```python
from build123d import *

# Parameters (mm, degrees)
F0_W     = 50.800353
F0_H     = 44.45
F1_DEPTH = 5


# Not quite as in the source:
# - ends of sketch curves that miss each other by under 0.0002 mm in the source are joined


with BuildPart() as f1:
    # F0 (on Front) → F1 (new body)
    with BuildSketch(Plane.XZ):
        with Locations((5e-07, 0)):
            Rectangle(F0_W, F0_H)
        with BuildLine():
            add(Edge.make_bspline(
                [(-7.08854, -11.336161), (-7.08854, -10.361789), (-7.878409, -9.572272), (-8.852429, -9.572272)],
                knots=[0, 0, 0, 0, 1, 1, 1, 1], degree=3))
            Line((-7.08854, -11.336161), (-7.08854, -15.052322))
            add(Edge.make_bspline(
                [(-8.852429, -16.816211), (-7.878409, -16.816211), (-7.08854, -16.026695), (-7.08854, -15.052322)],
                knots=[0, 0, 0, 0, 1, 1, 1, 1], degree=3))
            Line((-8.852429, -16.816211), (-16.378237, -16.816211))
            add(Edge.make_bspline(
                [(-18.142126, -15.052322), (-18.142126, -16.026695), (-17.352257, -16.816211), (-16.378237, -16.816211)],
                knots=[0, 0, 0, 0, 1, 1, 1, 1], degree=3))
            Line((-18.142126, -15.052322), (-18.142126, -11.336161))
            add(Edge.make_bspline(
                [(-16.378237, -9.572272), (-17.352257, -9.572272), (-18.142126, -10.361789), (-18.142126, -11.336161)],
                knots=[0, 0, 0, 0, 1, 1, 1, 1], degree=3))
            Line((-16.378237, -9.572272), (-8.852429, -9.572272))
        make_face(mode=Mode.SUBTRACT)
        with BuildLine():
            Line((-1.5500305536, -19.2250000002), (-1.5500305536, -8.1871465892))
            ThreePointArc((-1.5500305536, -8.1871465892), (-1.5500734508, -8.1804888446), (-1.55008775, -8.1738309772))
            ThreePointArc((-1.55008775, -8.1738309772), (-9.17611e-05, -6.6238309772), (1.54991225, -8.173822955))
            Line((1.54991225, -8.173822955), (1.5499694464, -19.224991978))
            ThreePointArc((1.5499694464, -19.224991978), (-2.65425e-05, -20.7749959891), (-1.5500305536, -19.2250000002))
        make_face(mode=Mode.SUBTRACT)
        with BuildLine():
            add(Edge.make_bspline(
                [(-0.0001188036, 5.1738309774), (-2.8576188036, 5.1738309774), (-5.1743108036, 2.8571389774), (-5.1743108036, -8.0226e-06)],
                knots=[0, 0, 0, 0, 1, 1, 1, 1], degree=3))
            add(Edge.make_bspline(
                [(5.1737201964, -8.0226e-06), (5.1737201964, 2.8571389774), (2.8573811964, 5.1738309774), (-0.0001188036, 5.1738309774)],
                knots=[0, 0, 0, 0, 1, 1, 1, 1], degree=3))
            add(Edge.make_bspline(
                [(-0.0001188036, -5.1742000226), (2.8573811964, -5.1742000226), (5.1737201964, -2.8578610226), (5.1737201964, -8.0226e-06)],
                knots=[0, 0, 0, 0, 1, 1, 1, 1], degree=3))
            add(Edge.make_bspline(
                [(-5.1743108036, -8.0226e-06), (-5.1743108036, -2.8578610226), (-2.8576188036, -5.1742000226), (-0.0001188036, -5.1742000226)],
                knots=[0, 0, 0, 0, 1, 1, 1, 1], degree=3))
        make_face(mode=Mode.SUBTRACT)
        with BuildLine():
            Line((-22.400176, 1.55), (-8.1743108036, 1.55))
            ThreePointArc((-8.1743108036, 1.55), (-6.624368, 0), (-8.174368, -1.55))
            Line((-8.174368, -1.55), (-22.400176, -1.55))
            ThreePointArc((-22.400176, -1.55), (-23.950176, 0), (-22.400176, 1.55))
        make_face(mode=Mode.SUBTRACT)
        with BuildLine():
            add(Edge.make_bspline(
                [(-12.941829, 20.343636), (-14.143743, 20.343636), (-15.117409, 19.369616), (-15.117409, 18.168055)],
                knots=[0, 0, 0, 0, 1, 1, 1, 1], degree=3))
            add(Edge.make_bspline(
                [(-10.766601, 18.168055), (-10.766601, 19.369616), (-11.740621, 20.343636), (-12.941829, 20.343636)],
                knots=[0, 0, 0, 0, 1, 1, 1, 1], degree=3))
            add(Edge.make_bspline(
                [(-12.941829, 15.992828), (-11.740621, 15.992828), (-10.766601, 16.966847), (-10.766601, 18.168055)],
                knots=[0, 0, 0, 0, 1, 1, 1, 1], degree=3))
            add(Edge.make_bspline(
                [(-15.117409, 18.168055), (-15.117409, 16.966847), (-14.143743, 15.992828), (-12.941829, 15.992828)],
                knots=[0, 0, 0, 0, 1, 1, 1, 1], degree=3))
        make_face(mode=Mode.SUBTRACT)
        with BuildLine():
            Line((-1.5500305536, 8.1871465892), (-1.5500305536, 19.2250000002))
            ThreePointArc((-1.5500305536, 19.2250000002), (-2.65425e-05, 20.7749959891), (1.5499694464, 19.224991978))
            Line((1.5499694464, 19.224991978), (1.54991225, 8.1738309772))
            ThreePointArc((1.54991225, 8.1738309772), (-9.17611e-05, 6.6238309772), (-1.55008775, 8.1738309772))
            Line((-1.55008775, 8.1738309772), (-1.5500305536, 8.1871465892))
        make_face(mode=Mode.SUBTRACT)
        with BuildLine():
            Line((8.1743108036, 1.55), (22.400176, 1.55))
            ThreePointArc((22.400176, 1.55), (23.950176, 0), (22.400176, -1.55))
            Line((22.400176, -1.55), (8.1743108036, -1.55))
            ThreePointArc((8.1743108036, -1.55), (6.624368, 0), (8.1743108036, 1.55))
        make_face(mode=Mode.SUBTRACT)
        with BuildLine():
            add(Edge.make_bspline(
                [(12.94571, 20.343636), (11.743796, 20.343636), (10.770129, 19.369616), (10.770129, 18.168055)],
                knots=[0, 0, 0, 0, 1, 1, 1, 1], degree=3))
            add(Edge.make_bspline(
                [(15.121291, 18.168055), (15.121291, 19.369616), (14.146918, 20.343636), (12.94571, 20.343636)],
                knots=[0, 0, 0, 0, 1, 1, 1, 1], degree=3))
            add(Edge.make_bspline(
                [(12.94571, 15.992828), (14.146918, 15.992828), (15.121291, 16.966847), (15.121291, 18.168055)],
                knots=[0, 0, 0, 0, 1, 1, 1, 1], degree=3))
            add(Edge.make_bspline(
                [(10.770129, 18.168055), (10.770129, 16.966847), (11.743796, 15.992828), (12.94571, 15.992828)],
                knots=[0, 0, 0, 0, 1, 1, 1, 1], degree=3))
        make_face(mode=Mode.SUBTRACT)
    extrude(amount=F1_DEPTH)


solid = f1.part
```
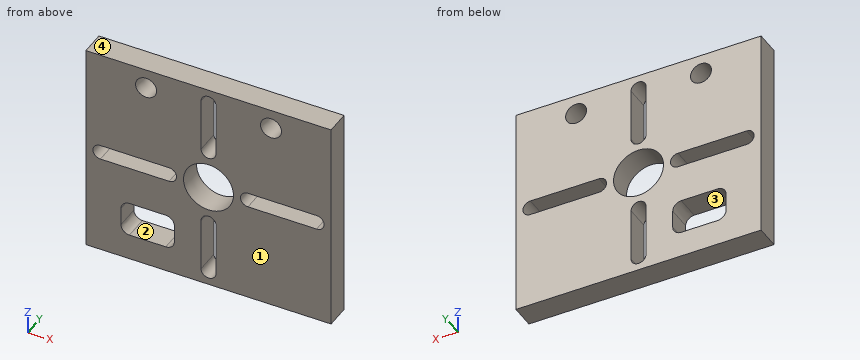
Work out the finished part from the listing and answer in its coordinate system (mm). Face numbers are marked on the shaded views. A direction names the side the tool comes from. Coordinates: 2 decimals unless noted, no trailing zeros. Write each loop counter-clockwise with the first axis right and the second up, starting at its lowest first coordinate (ties: lowest second). Pieces come first, ordered by that corner, then holes. Notation, with made-up numbers: (86.5, 60.5) - (139.5, 60.5) arc R12 ccw to (139.5, 73.5) - close; hole circle Ø9 at (-29, 52). An arc over 180 degrees is marked (long way). Answer as a JSON object with one key per item and string values.
Q1. Consider L1, parallel to X at y = -3.3, z = -13; L2, parallel to X at y = -1.45, z = 11.5; L3, parallel to Z at x = -21.5, y = -3.4 (3 decimals). Determine where each line is inside the solid, lowest interval first. Write a range as from..to.
Results list:
{"L1": "x = -25.4..-18.14, -7.09..-1.55, 1.55..25.4", "L2": "x = -25.4..-1.55, 1.55..25.4", "L3": "z = -22.225..-1.55, 1.55..22.225"}
Q2. Find section C-C (z = -12). Write down the section's boundary in (x, y), plus the area to 3 significant figures.
Results list:
{"outline": "(-25.4, -5) - (-18.14, -5) - (-18.14, 0) - (-25.4, 0) - close; (-7.09, -5) - (-1.55, -5) - (-1.55, 0) - (-7.09, 0) - close; (1.55, -5) - (25.4, -5) - (25.4, 0) - (1.55, 0) - close", "area": "183 mm^2"}
Q3. For a pull along X with two mould halves and no side action, classify the marked faces 1 and 2 as pulls with the +X half, pulls with the -X half, needs draft (parallel to the pull), parting line crosses it, or undercut.
Results list:
{"face 1": "needs draft", "face 2": "undercut"}
Q4. Find section D-D (y = -3.15). State how many separate pieces and enclosed holes the cut face has, plus the area to 3 significant figures.
Results list:
{"separate pieces": "1", "enclosed holes": "8", "area": "1,880 mm^2"}
Q5. Find section A-A (x = -10). Write down the section's boundary in (y, z) (3 decimals), plus the area to 3 significant figures.
Results list:
{"outline": "(-5, -22.225) - (0, -22.225) - (0, -16.816) - (-5, -16.816) - close; (-5, -9.572) - (0, -9.572) - (0, -1.55) - (-5, -1.55) - close; (-5, 1.55) - (0, 1.55) - (0, 22.225) - (-5, 22.225) - close", "area": "171 mm^2"}
Q6. Find section B-B (x = 10). Write down the section's boundary in (y, z) (3 decimals), plus the area to 3 significant figures.
Results list:
{"outline": "(-5, -22.225) - (0, -22.225) - (0, -1.55) - (-5, -1.55) - close; (-5, 1.55) - (0, 1.55) - (0, 22.225) - (-5, 22.225) - close", "area": "207 mm^2"}
Q7. Which of the six approach directions +Z, -Z, +X, -X, +Y, -Y give full straight-line access (tool end or side, diameter ignored) to the marked faces 3 and 4?
Results list:
{"face 3": "+Y, -Y", "face 4": "+Z, +X, -X, +Y, -Y"}
